The drawing under review shows one solid part. Ordinate dimensions are in mm from its lowest x, y, z. A direction names the side the tool comes from. Round coordinates to 2 decimals unless told otherwise and drop trailing zeros. Order: outer loops, then holes, each group sorted by start corner. A loop starts at its lowest first (then second) coordinate and runs counter-clockwise, first axis right, second up. Notation, with made-up numbers: (-7, 36) -> (46, 36) arc R34 ccw to (46, 68) -> close; hole circle Ø5 at (59.5, 70). An arc over 180 degrees is marked (long way). Use a Markdown table: item, result. Add a question column.
1) Clearance check with flat-ended pins moving along their axes: P1, Ø11, axis at x = 130.5, z = 3, coming from the -Y side; P2, Ø3, axis at x = 31, y = 62.5, coming from the +Z side; P3, Ø1.5, axis at x = 89.5, z = 45, coming from the +Y side. State where each tip first meets the part, or that it passes through.
2) Machinability: for the marked faces 1 and 2, which of the approach directions +Z, -Z, +X, -X, +Y, -Y give a long, thin tool a straight path to every point of the face, cutting with its end or side? Answer none if there is none.
3) Draft analysis for pull direction Z (two halves, no side actions). For the marked faces 3, 4, 5 and 6, state which applies: pulls with the +Z half, pulls with the -Z half, needs draft (parallel to the pull), parting line crosses it, or undercut.
4) Wall thickness on line 1 along X through (y, z) = (53.5, 6); line 2 along Z through (x, y) = (238, 23); line 3 along Y through (x, z) = (53.5, 30.5): over which ranges is each line inside the solid? List them lowest first. Write a range as [from, to].
5) Consider section C-C (y = 24). State the section outline as (x, z) points.
6) Consider section A-A (z = 26). State the section outline as (x, y) points, plus the area to 3 significant figures.
7) Consider section D-D (x = 226.5). State the section outline as (y, z) points, plus the area to 3 significant figures.
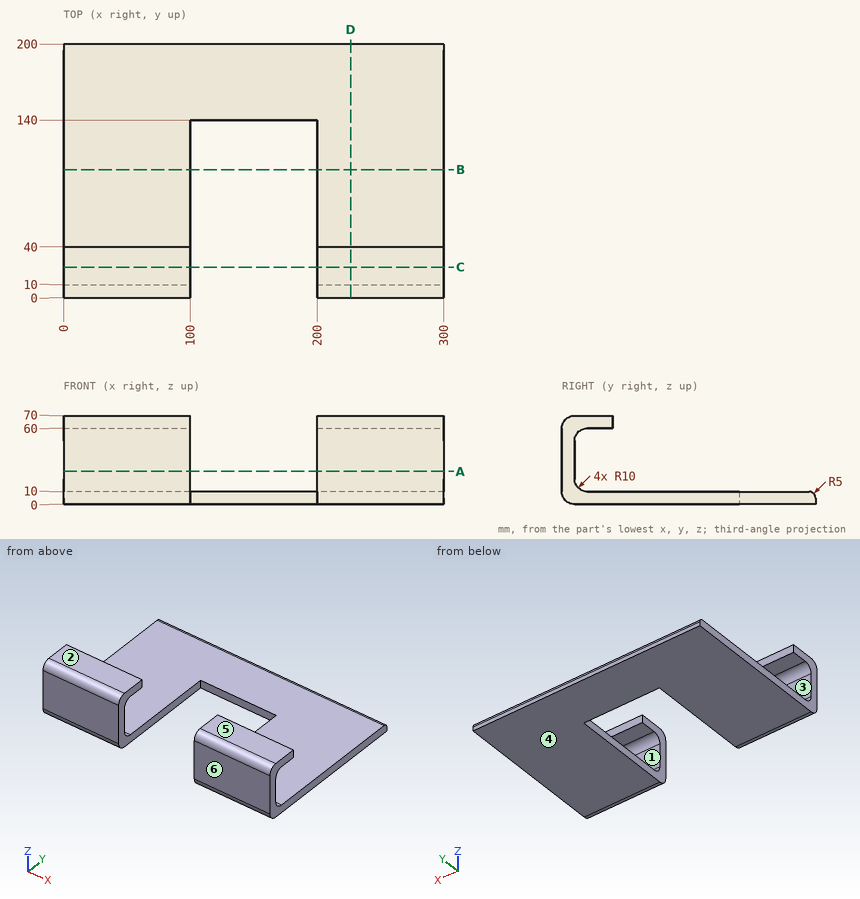
Results list:
| question | item | result |
|---|---|---|
| 1 | P1 | y = 140 |
| 1 | P2 | z = 10 |
| 1 | P3 | y = 10 |
| 2 | face 1 | +X, -X, +Y |
| 2 | face 2 | +Z, +X, -X, +Y, -Y |
| 3 | face 3 | undercut |
| 3 | face 4 | pulls with the -Z half |
| 3 | face 5 | pulls with the +Z half |
| 3 | face 6 | needs draft |
| 4 | line 1 | [0, 100], [200, 300] |
| 4 | line 2 | [0, 10], [60, 70] |
| 4 | line 3 | [0, 10] |
| 5 | outline | (0, 0) -> (100, 0) -> (100, 10) -> (0, 10) -> close; (0, 60) -> (100, 60) -> (100, 70) -> (0, 70) -> close; (200, 0) -> (300, 0) -> (300, 10) -> (200, 10) -> close; (200, 60) -> (300, 60) -> (300, 70) -> (200, 70) -> close |
| 6 | outline | (0, 0) -> (100, 0) -> (100, 10) -> (0, 10) -> close; (200, 0) -> (300, 0) -> (300, 10) -> (200, 10) -> close |
| 6 | area | 2,000 mm2 |
| 7 | outline | (0, 10) arc R10 ccw to (10, 0) -> (200, 0) -> (200, 5) arc R5 ccw to (195, 10) -> (20, 10) arc R10 cw to (10, 20) -> (10, 50) arc R10 cw to (20, 60) -> (40, 60) -> (40, 70) -> (10, 70) arc R10 ccw to (0, 60) -> close |
| 7 | area | 2,890 mm2 |
